Autodesk Inventor part; units mm, degrees
ref_plane "YZ Plane" through (0, 0, 0) normal (1, 0, 0) x (0, 1, 0)
ref_plane "XZ Plane" through (0, 0, 0) normal (0, 1, 0) x (-1, 0, 0)
ref_plane "XY Plane" through (0, 0, 0) normal (0, 0, 1) x (1, 0, 0)
sketch "Sketch1" plane through (0, 0, 0) normal (0, 0, 1) x (1, 0, 0)
  circle A0 centre (0, 0) radius 34
  circle A1 centre (0, 0) radius 4
  circle A2 centre (-18, 0) radius 3.175
  circle A3 centre (18, 0) radius 3.175
  dimension "d0" = 68
  dimension "d1" = 8
  dimension "d2" = 18
  dimension "d3" = 18
  dimension "d4" = 6.35
extrude "Extrusion1" add sketch "Sketch1" against normal blind 100 contours A0 | A1 | A2 | A3
extrude "Extrusion2" cut sketch "Sketch1" against normal blind 25.4 contours A2 | A3
extrude "Extrusion3" add sketch "Sketch1" along normal blind 28 contours A1
fillet "Fillet1" radius 3.175 2 edges at (-34, 0, 0) (-34, 0, -100)
equation "\"d3\" = d2"
properties part number "DC Brush Motor 24V 150W High Speed Motor with Belt Pulley for DIY Generator Electric Vehicle Motor"
The model under review builds one solid part; all positions refer to its coordinate system, in mm. A direction names the side the tool comes from. Give positions to 0.01 mm unless a question says otherwise; leave off trailing zeros. Write each loop counter-clockwise with the first axis right and the second up, starting at its lowest first coordinate (ties: lowest second). Pieces come first, ordered by that corner, then holes. Notation, with made-up numbers: (69, -5) - (118, -5) arc R28 cw to (118, 31) - close; hole circle Ø8 at (48.5, 39). An arc over 180 degrees is marked (long way). Answer in a Markdown table with one row per item. Add a question column.
1. Draft analysis for pull direction X (two halves, no side actions). For faces 1 (the flat face through (0, 0, -100)), 2 (the cylindrical face through (18.28, 28.67, -49.34)), 3 (the cylindrical face through (14.83, 0.14, -12.52)), 4 (the flat face through (18, 0, -25.4)), state which applies: +X half, -X half, draft (parallel to the pull), parting line (faces both ways), or undercut.
2. We need section D-D on z = -46. Write out the cut boundary in (x, y).
3. We need section C-C on z = -19. Write out the cut boundary in (x, y) (3 decimals), then the cut area to 3 significant figures.
4. Tool access review of faces 5 (the flat face through (0, 0, 28)), 6 (the cylindrical face through (-0.867, 3.905, 13.804)): name each direction out of +Z, -Z, +X, -X, +Y, -Y from which nothing blocks a thin tool from reaching the whole face with its end or side.
5. We need section A-A on x = 0. Write out the cut boundary in (y, z) (3 decimals), then the cut area to 3 significant figures.
6. We need section B-B on y = 0. Write out the cut boundary in (x, z) (3 decimals).
7. Insertion check: P1, Ø12, axis at x = 24.5, y = -6, coming from the +Z side; P2, Ø12, axis at y = -25, z = -48.5, coming from the +X side; P3, Ø2, axis at x = 13.5, z = -1, coming from the -Y side. Each pin has a flat end and moves straight along its axis. Give the tip position at first contact, or say it passes through.
8. Wall thickness on line 1 along Z through (x, y) = (11.5, 13.5); line 2 along X through (y, z) = (-1, -79); line 3 along Y through (x, z) = (-18, -9) (3 decimals): over which ranges is each line inside the solid? List them lowest first. Write a range as [from, to].
Ans:
| question | item | result |
|---|---|---|
| 1 | face 1 | draft |
| 1 | face 2 | parting line |
| 1 | face 3 | undercut |
| 1 | face 4 | undercut |
| 2 | outline | circle Ø68 at (0, 0) |
| 3 | outline | circle Ø68 at (0, 0); hole circle Ø6.35 at (-18, 0); hole circle Ø6.35 at (18, 0) |
| 3 | area | 3,570 mm^2 |
| 4 | face 5 | +Z, +X, -X, +Y, -Y |
| 4 | face 6 | +Z |
| 5 | outline | (-34, -96.825) arc R3.175 ccw to (-30.825, -100) - (30.825, -100) arc R3.175 ccw to (34, -96.825) - (34, -3.175) arc R3.175 ccw to (30.825, 0) - (4, 0) - (4, 28) - (-4, 28) - (-4, 0) - (-30.825, 0) arc R3.175 ccw to (-34, -3.175) - close |
| 5 | area | 7,020 mm^2 |
| 6 | outline | (-34, -96.825) arc R3.175 ccw to (-30.825, -100) - (30.825, -100) arc R3.175 ccw to (34, -96.825) - (34, -3.175) arc R3.175 ccw to (30.825, 0) - (21.175, 0) - (21.175, -25.4) - (14.825, -25.4) - (14.825, 0) - (4, 0) - (4, 28) - (-4, 28) - (-4, 0) - (-14.825, 0) - (-14.825, -25.4) - (-21.175, -25.4) - (-21.175, 0) - (-30.825, 0) arc R3.175 ccw to (-34, -3.175) - close |
| 7 | P1 | stops at z = 0 |
| 7 | P2 | stops at x = 28.2 |
| 7 | P3 | stops at y = -31.12 |
| 8 | line 1 | z = [-100, 0] |
| 8 | line 2 | x = [-33.99, 33.99] |
| 8 | line 3 | y = [-28.844, -3.175], [3.175, 28.844] |
